The drawing under review shows one solid part. Ordinate dimensions are in mm from its lowest x, y, z. Give positions to 0.01 mm unless a question says otherwise; leave off trailing zeros. Loops run counter-clockwise (first coordinate to the right, second up) from the corner with the lowest first, then second, coordinate; pieces in that order, holes last. Notation, with made-up numbers: M -10.75,-25.5 L 38.25,-25.5 A32 ccw 38.25,0.5 Z; hole C 45.25,69 d8. An arc over 180 degrees is marked long. Answer as CSV lines item,"result".
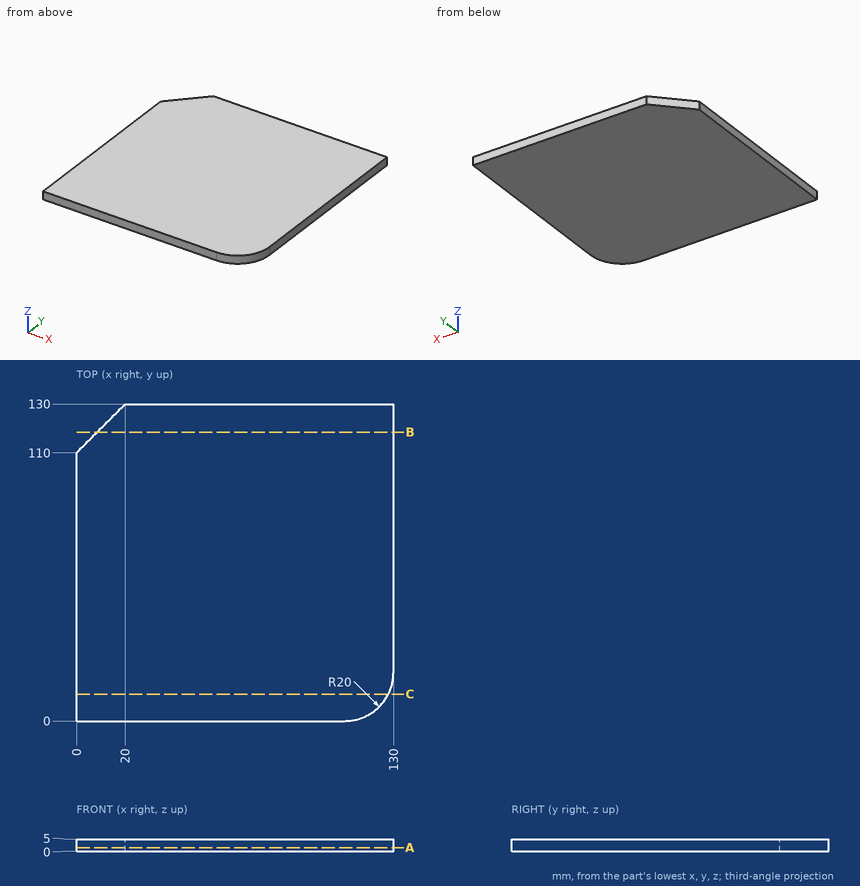
1. We need section A-A, the plane z = 1.45. Write out the cut boundary in (x, y), plus the area to 3 significant figures.
Answer block:
outline,"M 0,0 L 110,0 A20 ccw 130,20 L 130,130 L 20,130 L 0,110 Z"
area,"16,600 mm²"
2. To check wall thickness, follow L1, parallel to Y at x = 118, z = 1.6; L2, parallel to Y at x = 114, z = 2.25; L3, parallel to X at y = 119.5, z = 2.25. State the ranges of each line that lie inside material, in increasing order. Write a range as [from, to].
Answer block:
L1,"[1.67, 130]"
L2,"[0.4, 130]"
L3,"[9.5, 130]"
3. For P1, Ø1, axis at y = 112, z = 1.5, coming from the -X side, flat-tipped, find the tip position at first contact; note if it passes through.
Answer block:
P1,"x = 1.5"
4. We need section B-B, the plane y = 118.5. Write out the cut boundary in (x, z).
Answer block:
outline,"M 8.5,0 L 130,0 L 130,5 L 8.5,5 Z"
5. We need section C-C, the plane y = 11. Write out the cut boundary in (x, z), plus the area to 3 significant figures.
Answer block:
outline,"M 0,0 L 127.86,0 L 127.86,5 L 0,5 Z"
area,"639 mm²"
